Input: dimensioned drawing with shaded views. Units: mm. Origin: part minimum x, y, z. Round coordinates to 2 decimals unless told otherwise and drop trailing zeros. Write each loop counter-clockwise with the first axis right and the second up, starting at its lowest first coordinate (ties: lowest second). Pieces come first, ordered by that corner, then holes. Notation, with made-up numbers: M -23,61 L 12,61 A29 ccw 12,89 Z; hole C 73.5,-19.75 d11. An arc over 180 degrees is marked long. Answer in a Markdown table with one row per item. Add a question column.
Item 1: Cut plane B-B on x = 13.9. Return loops of the section in (y, z) (3 decimals), and give its area (3 significant figures).
Item 2: Cut plane D-D on z = 4. Return loops of the section in (x, y) (3 decimals), and give its area (3 significant figures).
Item 3: Mould query, pull axis Y, two halves, no side actions, for the marked faces 1, 2 and 3. Classes: released by +Y, released by -Y, zero draft, split by the parting line, or undercut.
Item 4: Cut plane A-A on y = 13.9. Return loops of the section in (x, z) (3 decimals), and give its area (3 significant figures).
Item 5: Material intervals for probe 1 along Y at (x, z) = (13.9, 3.5) (3 decimals); probe 2 along Y at (x, z) = (15, 1.25); probe 3 along X at (y, z) = (14.5, 2.5), sorted ascending.
Item 6: Cut plane C-C on z = 5.5. Return loops of the section in (x, y) (3 decimals), and give its area (3 significant figures).
Item 7: Contact query for flat-ended pins moving along their axis: pin 1 (1 mm diameter, centred on y = 6.5, z = 1, fed in from -X); pin 2 (2 mm diameter, centred on y = 12.5, z = 4.5, fed in from +X); pin 3 (1.5 mm diameter, centred on x = 7.5, z = 4, fed in from +Y). Output: stop coordinate, or through.
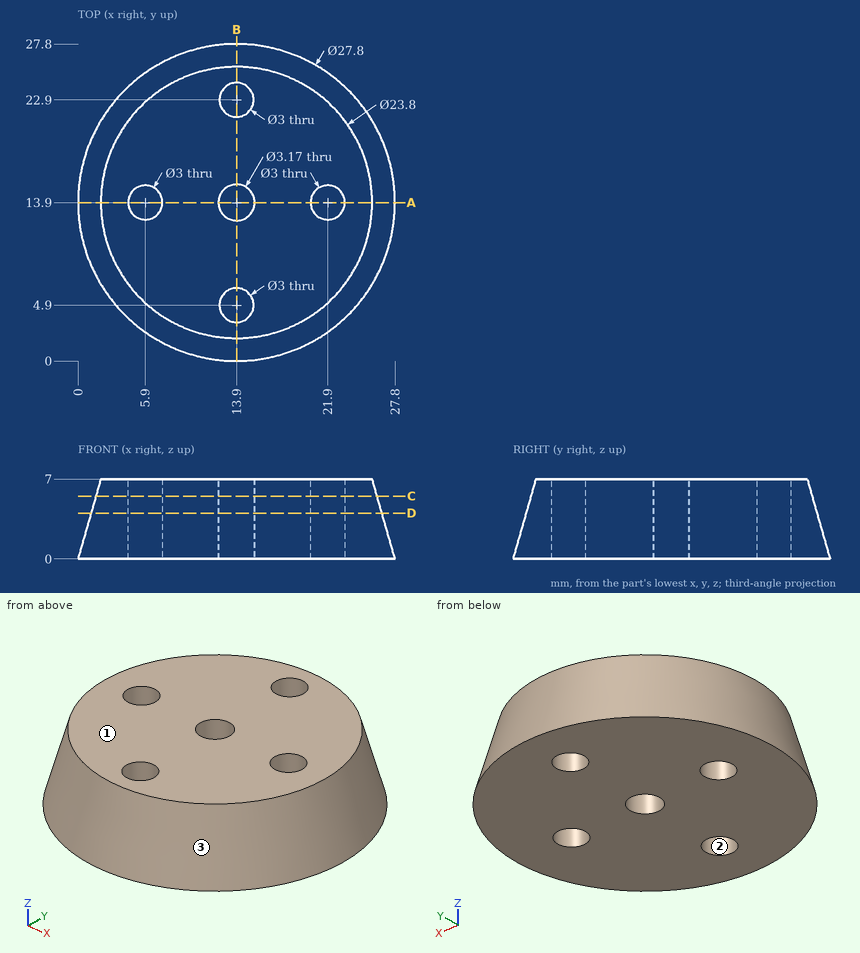
Results below:
| question | item | result |
|---|---|---|
| 1 | outline | M 0,0 L 3.4,0 L 3.4,7 L 2,7 Z; M 6.4,0 L 12.315,0 L 12.315,7 L 6.4,7 Z; M 15.485,0 L 21.4,0 L 21.4,7 L 15.485,7 Z; M 24.4,0 L 27.8,0 L 25.8,7 L 24.4,7 Z |
| 1 | area | 116 mm2 |
| 2 | outline | C 13.9,13.9 d25.514; hole C 5.9,13.9 d3; hole C 13.9,13.9 d3.17; hole C 13.9,4.9 d3; hole C 13.9,22.9 d3; hole C 21.9,13.9 d3 |
| 2 | area | 475 mm2 |
| 3 | face 1 | zero draft |
| 3 | face 2 | undercut |
| 3 | face 3 | split by the parting line |
| 4 | outline | M 0,0 L 4.4,0 L 4.4,7 L 2,7 Z; M 7.4,0 L 12.315,0 L 12.315,7 L 7.4,7 Z; M 15.485,0 L 20.4,0 L 20.4,7 L 15.485,7 Z; M 23.4,0 L 27.8,0 L 25.8,7 L 23.4,7 Z |
| 4 | area | 116 mm2 |
| 5 | probe 1 | 1 to 3.4, 6.4 to 12.315, 15.485 to 21.4, 24.4 to 26.8 |
| 5 | probe 2 | 0.4 to 3.88, 5.92 to 12.76, 15.04 to 21.88, 23.92 to 27.4 |
| 5 | probe 3 | 0.73 to 4.53, 7.27 to 12.43, 15.37 to 20.53, 23.27 to 27.07 |
| 6 | outline | C 13.9,13.9 d24.657; hole C 5.9,13.9 d3; hole C 13.9,13.9 d3.17; hole C 13.9,4.9 d3; hole C 13.9,22.9 d3; hole C 21.9,13.9 d3 |
| 6 | area | 441 mm2 |
| 7 | pin 1 | x = 2.12 |
| 7 | pin 2 | x = 26.74 |
| 7 | pin 3 | y = 25.41 |
